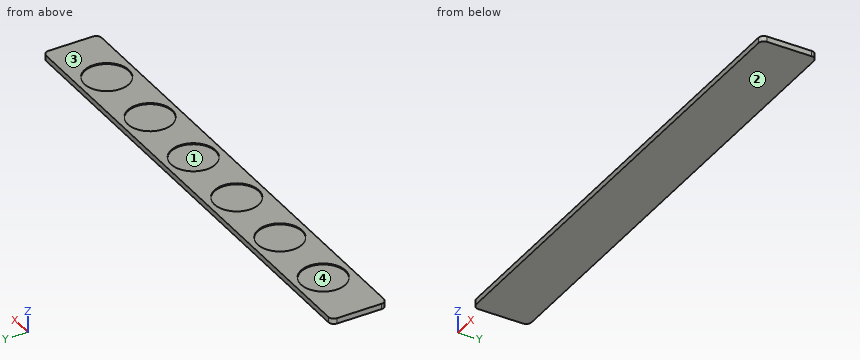
```python
from build123d import *

# Parameters (mm, degrees)
SKETCH_W            = 440
SKETCH_H            = 50
PAD_DEPTH           = 5
SKETCH001_R         = 20
POCKET_DEPTH        = 1
LINEARPATTERN_COUNT = 6
LINEARPATTERN_PITCH = 66
FILLET_R            = 5
FILLET001_R         = 5


with BuildPart() as part:
    # Sketch → Pad (new body)
    with BuildSketch(Plane.XY):
        with Locations((163.979408, 5.129884)):
            Rectangle(SKETCH_W, SKETCH_H)
    extrude(amount=PAD_DEPTH)

    # Sketch001 → Pocket (cut)
    with BuildSketch(Plane.XY.offset(5)):
        with Locations((-1.020592, 5.129884)):
            Circle(SKETCH001_R)
    pocket = extrude(amount=-POCKET_DEPTH, mode=Mode.SUBTRACT)

    # LinearPattern: Pocket ×6
    with Locations(*[(i * LINEARPATTERN_PITCH, 0, 0) for i in range(1, LINEARPATTERN_COUNT)]):
        add(pocket, mode=Mode.SUBTRACT)

    # Fillet
    fillet_edges = [part.edges().sort_by_distance(p)[0] for p in [
        (-56.020592, 30.129884, 2.5),
        (383.979408, -19.870116, 2.5),
        (383.979408, 30.129884, 2.5),
    ]]
    fillet(fillet_edges, radius=FILLET_R)

    # Fillet001
    fillet001_edges = [part.edges().sort_by_distance(p)[0] for p in [
        (-56.020592, -19.870116, 2.5),
    ]]
    fillet(fillet001_edges, radius=FILLET001_R)


solid = part.part
```
Verification items for the finished model (mm, model axes). Face numbers are marked on the shaded views. A direction names the side the tool comes from. Coordinates: 2 decimals unless noted, no trailing zeros. Loops run counter-clockwise (first coordinate to the right, second up) from the corner with the lowest first, then second, coordinate; pieces in that order, holes last. Notation, with made-up numbers: (16, 38) -> (37, 38) arc R10 ccw to (37, 52) -> close; hole circle Ø2 at (44.25, -4.75). An arc over 180 degrees is marked (long way). Answer in a Markdown table with one row per item.
1) Access from +Z, -Z, +X, -X, +Y, -Y to the whole of each face (thin tool, end or side, straight path). Record for the marked faces 1 and 2.
The answers:
| item | result |
|---|---|
| face 1 | +Z |
| face 2 | -Z, +X, -X, +Y, -Y |
2) Scan lines: line 1 along Z through (x, y) = (0, 25); line 2 along Y through (x, z) = (326, 4.3); line 3 along X through (y, z) = (-17, 2.4). Record each from-to range of solid material in increasing order. Write a range as from..to.
The answers:
| item | result |
|---|---|
| line 1 | z = 0..4 |
| line 2 | y = -19.87..-14.65, 24.91..30.13 |
| line 3 | x = -55.54..383.5 |
3) Section check A-A (x = 78). Record the cut outline in (y, z).
The answers:
| item | result |
|---|---|
| outline | (-19.87, 0) -> (30.13, 0) -> (30.13, 5) -> (20.31, 5) -> (20.31, 4) -> (-10.05, 4) -> (-10.05, 5) -> (-19.87, 5) -> close |
4) Draft check along X on the marked faces 3 and 4. Enter one of: released by +X, released by -X, zero draft, split by the parting line, or undercut.
The answers:
| item | result |
|---|---|
| face 3 | zero draft |
| face 4 | undercut |
5) Section check B-B (y = -2). Record the cut outline in (x, z), and give its area (3 significant figures).
The answers:
| item | result |
|---|---|
| outline | (-56.02, 0) -> (383.98, 0) -> (383.98, 5) -> (347.67, 5) -> (347.67, 4) -> (310.29, 4) -> (310.29, 5) -> (281.67, 5) -> (281.67, 4) -> (244.29, 4) -> (244.29, 5) -> (215.67, 5) -> (215.67, 4) -> (178.29, 4) -> (178.29, 5) -> (149.67, 5) -> (149.67, 4) -> (112.29, 4) -> (112.29, 5) -> (83.67, 5) -> (83.67, 4) -> (46.29, 4) -> (46.29, 5) -> (17.67, 5) -> (17.67, 4) -> (-19.71, 4) -> (-19.71, 5) -> (-56.02, 5) -> close |
| area | 1,980 mm2 |
6) Section check C-C (x = 255). Record the cut outline in (y, z), and give its area (3 significant figures).
The answers:
| item | result |
|---|---|
| outline | (-19.87, 0) -> (30.13, 0) -> (30.13, 5) -> (23.47, 5) -> (23.47, 4) -> (-13.21, 4) -> (-13.21, 5) -> (-19.87, 5) -> close |
| area | 213 mm2 |
7) Depth check by flat-ended pin: P1, Ø8, axis at x = 228.5, y = 23.5, coming from the -Z side; P2, Ø24, axis at x = 64.98, y = 5.13, coming from the +Z side. Enter the tip coordinate at first touch or a pass-through.
The answers:
| item | result |
|---|---|
| P1 | stops at z = 0 |
| P2 | stops at z = 4 |
